The listing builds one solid part. Answer for the finished solid, in the listing's coordinates (mm). Give positions to 0.01 mm unless a question says otherwise; leave off trailing zeros. Write each loop counter-clockwise with the first axis right and the second up, starting at its lowest first coordinate (ties: lowest second). Pieces come first, ordered by that corner, then holes. Notation, with made-up numbers: (76.5, 63) -> (86.5, 63) arc R26 ccw to (86.5, 91) -> close; hole circle Ø9 at (-10.75, -31.75). An arc over 180 degrees is marked (long way). Write each question's results on one line, items separated by ' | '. Start each with the question number.
from build123d import *

# Parameters (mm, degrees)
BOSS_EXTRUDE1_DEPTH     = 1.25
FILLET1_R               = 10
FILLET2_R               = 1
FILLET3_R               = 1
SKETCH2_R               = 1.25
CUT_EXTRUDE1_DEPTH      = 3.5
LPATTERN1_COUNT         = 7
LPATTERN1_PITCH         = 6
SKETCH3_R               = 0.75
CUT_EXTRUDE2_DEPTH      = 10.0000001
CUT_EXTRUDE2_DEPTH_BACK = 10


with BuildPart() as part:
    # Sketch1 → Boss-Extrude1 (new body, symmetric)
    with BuildSketch(Plane(origin=(0, 0, 0), x_dir=(1, 0, 0), z_dir=(0, 1, 0))):
        Polygon((-59.638554217, 9), (-59.638554217, -9), (50.361445783, -9), (60.361445783, 0), (50.361445783, 9), align=None)
    extrude(amount=BOSS_EXTRUDE1_DEPTH, both=True)

    # Fillet1
    fillet1_edges = [part.edges().sort_by_distance(p)[0] for p in [
        (50.361445783, 0, 9),
        (50.361445783, 0, -9),
    ]]
    fillet(fillet1_edges, radius=FILLET1_R)

    # Fillet2
    fillet2_edges = [part.edges().sort_by_distance(p)[0] for p in [
        (60.361445783, 0, 0),
    ]]
    fillet(fillet2_edges, radius=FILLET2_R)

    # Fillet3
    fillet3_edges = [part.edges().sort_by_distance(p)[0] for p in [
        (-59.638554217, 1.25, 0),
        (-6.557234243, -1.25, -9),
        (-6.557234243, 1.25, -9),
        (56.374648223, -1.25, 3.588117804),
        (50.106723403, -1.25, 8.336204117),
        (50.106723403, -1.25, -8.336204117),
        (-6.557234243, 1.25, 9),
        (56.374648223, 1.25, 3.588117804),
        (50.106723403, 1.25, 8.336204117),
        (50.106723403, 1.25, -8.336204117),
        (56.374648223, -1.25, -3.588117804),
        (56.374648223, 1.25, -3.588117804),
        (59.866598667, -1.25, 0),
        (59.866598667, 1.25, 0),
        (-6.557234243, -1.25, 9),
        (-59.638554217, -1.25, 0),
    ]]
    fillet(fillet3_edges, radius=FILLET3_R)

    # Sketch2 → Cut-Extrude1 (cut, through all)
    with BuildSketch(Plane(origin=(0, 1.25, 0), x_dir=(1, 0, 0), z_dir=(0, 1, 0))):
        with Locations((42.866598667, 0)):
            Circle(SKETCH2_R)
    cut_extrude1 = extrude(amount=-CUT_EXTRUDE1_DEPTH, mode=Mode.SUBTRACT)

    # LPattern1: Cut-Extrude1 ×7
    with Locations(*[(-i * LPATTERN1_PITCH, 0, 0) for i in range(1, LPATTERN1_COUNT)]):
        add(cut_extrude1, mode=Mode.SUBTRACT)

    # Sketch3 → Cut-Extrude2 (cut, two sides)
    with BuildSketch(Plane.XY) as cut_extrude2_sk:
        with Locations((-58.019579169, 0)):
            Circle(SKETCH3_R)
    extrude(amount=CUT_EXTRUDE2_DEPTH, mode=Mode.SUBTRACT)
    extrude(cut_extrude2_sk.sketch, amount=-CUT_EXTRUDE2_DEPTH_BACK, mode=Mode.SUBTRACT)


solid = part.part
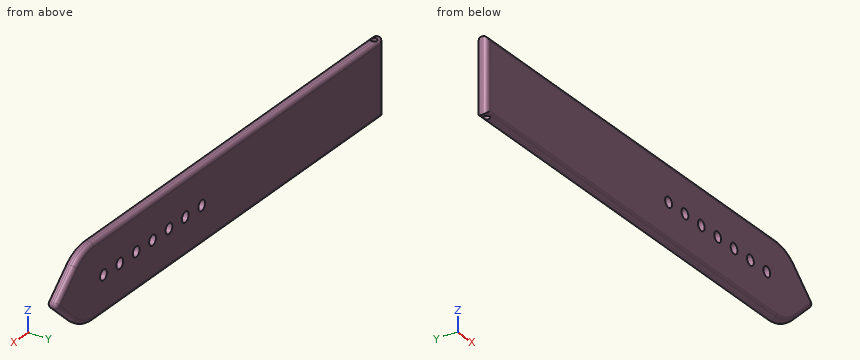
1. Section A-A (x = -33) is taken. Write down the section's boundary in (y, z), then the cut area to 3 significant figures.
2. This flat-tipped pin is pushed along its axis until it touches: pin 1 Ø1 at (y, z) = (-1, -2) entering from +X. Where does it stop, or does it pass through?
3. Consider probe 1 along Z at (x, y) = (-45, -0.3); probe 2 along Z at (x, y) = (26, 0.05); probe 3 along Z at (x, y) = (18, 0.95). Determine where each line is inside the solid, lowest interval first. Write a range as [from, to].
Results:
1) outline: (-1.25, -8) arc R1 ccw to (-0.25, -9) -> (0.25, -9) arc R1 ccw to (1.25, -8) -> (1.25, 8) arc R1 ccw to (0.25, 9) -> (-0.25, 9) arc R1 ccw to (-1.25, 8) -> close | area: 44.1 mm²
2) pin 1: stops at x = 58.42
3) probe 1: z = [-9, 9] | probe 2: z = [-9, -0.53], [0.53, 9] | probe 3: z = [-8.71, -0.9], [0.9, 8.71]
